from build123d import *
from OCP.BRepFilletAPI import BRepFilletAPI_MakeChamfer

# Parameters (mm, degrees)
EXTRUDE_1_DEPTH      = 1852
FILLET_1_R           = 5
CHAMFER_1_SIZE       = 2
CHAMFER_1_SIZE2      = 1.574468085
EXTRUDE_2_DEPTH      = 822
SKETCH_5_W           = 47
SKETCH_5_H           = 314
EXTRUDE_3_DEPTH      = 30
SKETCH_7_W           = 100
SKETCH_7_H           = 314
CUT_EXTRUDE_1_DEPTH  = 2
SKETCH_8_W           = 23
SKETCH_8_H           = 314
EXTRUDE_4_DEPTH      = 4
SKETCH_9_W           = 48
SKETCH_9_H           = 314
EXTRUDE_5_DEPTH      = 30
SKETCH_10_W          = 100
SKETCH_10_H          = 314
CUT_EXTRUDE_2_DEPTH  = 2
SKETCH_11_W          = 25
SKETCH_11_H          = 314
EXTRUDE_6_DEPTH      = 4
SKETCH_12_W          = 1742
SKETCH_12_H          = 169.004058013
CUT_EXTRUDE_3_DEPTH  = 80
SKETCH_13_W          = 822
SKETCH_13_H          = 239
CUT_EXTRUDE_4_DEPTH  = 5
SKETCH_14_W          = 736
SKETCH_14_H          = 219
CUT_EXTRUDE_5_DEPTH  = 71
SKETCH_15_R          = 45
CUT_EXTRUDE_6_DEPTH  = 1884.868315719
SKETCH_16_W          = 736
SKETCH_16_H          = 41
CUT_EXTRUDE_7_DEPTH  = 20
SKETCH_17_R          = 7.5
CUT_EXTRUDE_8_DEPTH  = 30
SKETCH_18_R          = 7.5
CUT_EXTRUDE_9_DEPTH  = 113
SKETCH_21_R          = 7.5
CUT_EXTRUDE_11_DEPTH = 111
SKETCH_23_R          = 7.5
CUT_EXTRUDE_12_DEPTH = 111


with BuildPart() as part:
    # 草图2 → 凸台-拉伸1 (new body)
    with BuildSketch(Plane(origin=(0, 0, 0), x_dir=(0, 0, -1), z_dir=(1, 0, 0))):
        Polygon((-76.260223553, 62.638496495), (-46.260223553, 62.638496495), (-46.260223553, 27.638496495), (36.739776447, 27.638496495), (36.739776447, -286.361503505), (-46.260223553, -286.361503505), (-46.260223553, -241.361503505), (-41.530493824, -239.739881883), (-43.152115445, -235.010152153), (-76.260223553, -246.361503505), (-76.260223553, -176.361503505), (-66.260223553, -176.361503505), (-66.260223553, -7.357445492), (-71.260223553, -7.357445492), (-71.260223553, -2.361503505), (-76.260223553, -2.361503505), align=None)
    extrude(amount=EXTRUDE_1_DEPTH)

    # 圆角1
    # the kernel refuses this fillet: 5 mm, written as the material it adds along each edge
    with BuildSketch(Plane(origin=(0, -2.361503505, 71.260223553), x_dir=(0, -1, 0), z_dir=(1, 0, 0))) as fillet_1_piece_1_section:
        with BuildLine():
            CenterArc((FILLET_1_R, -FILLET_1_R), FILLET_1_R, 90, 90)
            Line((0, -FILLET_1_R), (0, 0))
            Line((0, 0), (FILLET_1_R, 0))
        make_face()
    fillet_1_piece_1 = extrude(amount=1852, mode=Mode.PRIVATE)
    fillet_1_piece_1 = split(fillet_1_piece_1, bisect_by=Plane(origin=(926, -7.357445492, 72.392274368), z_dir=(0, 1, 0)), keep=Keep.TOP, mode=Mode.PRIVATE)
    add(fillet_1_piece_1)

    # 倒角1: one chamfer whose edges measure the first distance from different faces: ONE call of the kernel's chamfer builder (chamfer() names one face for all edges)
    chamfer_1_edges_1 = [part.edges().sort_by_distance(p)[0] for p in [
        (926, 62.638496495, 76.260223553),
        (926, -286.361503505, 46.260223553),
    ]]
    chamfer_1_edges_2 = [part.edges().sort_by_distance(p)[0] for p in [
        (926, -246.361503505, 76.260223553),
    ]]
    chamfer_1_side_2 = [part.faces().sort_by_distance(p)[0] for p in [
        (926, -211.361503505, 76.260223553),
    ]]
    chamfer_1 = BRepFilletAPI_MakeChamfer(part.part.solid().wrapped)
    for e in chamfer_1_edges_1:
        chamfer_1.Add(CHAMFER_1_SIZE, e.wrapped)
    for e in chamfer_1_edges_2:
        chamfer_1.Add(CHAMFER_1_SIZE, CHAMFER_1_SIZE2, e.wrapped, chamfer_1_side_2[0].wrapped)  # the first distance lies on this face
    add(Compound.cast(chamfer_1.Shape()), mode=Mode.REPLACE)

    # 草图4 → 凸台-拉伸2 (add)
    with BuildSketch(Plane(origin=(1337, 0, 0), x_dir=(0, 0, -1), z_dir=(1, 0, 0))):
        Polygon((36.739776447, 27.638496495), (56.739776447, 27.638496495), (56.739776447, 32.638496495), (71.739776447, 32.638496495), (71.739776447, 67.638496495), (111.739776447, 67.638496495), (111.739776447, -326.361503505), (71.739776447, -326.361503505), (71.739776447, -291.361503505), (56.739776447, -291.361503505), (56.739776447, -286.361503505), (36.739776447, -286.361503505), align=None)
    extrude(amount=-EXTRUDE_2_DEPTH)

    # 草图5 → 凸台-拉伸3 (add)
    with BuildSketch(Plane(origin=(0, 0, -36.739776447), x_dir=(-1, 0, 0), z_dir=(0, 0, -1))):
        with Locations((-1703.5, -129.361503505)):
            Rectangle(SKETCH_5_W, SKETCH_5_H)
    extrude(amount=EXTRUDE_3_DEPTH)

    # 草图7 → 切除-拉伸1 (cut)
    with BuildSketch(Plane(origin=(0, 0, -36.739776447), x_dir=(-1, 0, 0), z_dir=(0, 0, -1))):
        with Locations((-1510, -129.361503505)):
            Rectangle(SKETCH_7_W, SKETCH_7_H)
    extrude(amount=-CUT_EXTRUDE_1_DEPTH, mode=Mode.SUBTRACT)

    # 草图8 → 凸台-拉伸4 (add)
    with BuildSketch(Plane(origin=(0, 0, -36.739776447), x_dir=(-1, 0, 0), z_dir=(0, 0, -1))):
        with Locations((-1348.5, -129.361503505)):
            Rectangle(SKETCH_8_W, SKETCH_8_H)
    extrude(amount=EXTRUDE_4_DEPTH)

    # 草图9 → 凸台-拉伸5 (add)
    with BuildSketch(Plane(origin=(0, 0, -36.739776447), x_dir=(-1, 0, 0), z_dir=(0, 0, -1))):
        with Locations((-136, -129.361503505)):
            Rectangle(SKETCH_9_W, SKETCH_9_H)
    extrude(amount=EXTRUDE_5_DEPTH)

    # 草图10 → 切除-拉伸2 (cut)
    with BuildSketch(Plane(origin=(0, 0, -36.739776447), x_dir=(-1, 0, 0), z_dir=(0, 0, -1))):
        with Locations((-340, -129.361503505)):
            Rectangle(SKETCH_10_W, SKETCH_10_H)
    extrude(amount=-CUT_EXTRUDE_2_DEPTH, mode=Mode.SUBTRACT)

    # 草图11 → 凸台-拉伸6 (add)
    with BuildSketch(Plane(origin=(0, 0, -36.739776447), x_dir=(-1, 0, 0), z_dir=(0, 0, -1))):
        with Locations((-502.5, -129.361503505)):
            Rectangle(SKETCH_11_W, SKETCH_11_H)
    extrude(amount=EXTRUDE_6_DEPTH)

    # 草图12 → 切除-拉伸3 (cut)
    with BuildSketch(Plane.XY.offset(66.260223553)):
        with Locations((926, -91.859474499)):
            Rectangle(SKETCH_12_W, SKETCH_12_H)
    extrude(amount=-CUT_EXTRUDE_3_DEPTH, mode=Mode.SUBTRACT)

    # 草图13 → 切除-拉伸4 (cut)
    with BuildSketch(Plane(origin=(0, 0, -111.739776447), x_dir=(-1, 0, 0), z_dir=(0, 0, -1))):
        with Locations((-926, -125.861503505)):
            Rectangle(SKETCH_13_W, SKETCH_13_H)
    extrude(amount=-CUT_EXTRUDE_4_DEPTH, mode=Mode.SUBTRACT)

    # 草图14 → 切除-拉伸5 (cut)
    with BuildSketch(Plane(origin=(0, 0, -106.739776447), x_dir=(-1, 0, 0), z_dir=(0, 0, -1))):
        with Locations((-926, -125.861503505)):
            Rectangle(SKETCH_14_W, SKETCH_14_H)
    extrude(amount=-CUT_EXTRUDE_5_DEPTH, mode=Mode.SUBTRACT)

    # 草图15 → 切除-拉伸6 (cut, through all)
    with BuildSketch(Plane(origin=(0, 0, -35.739776447), x_dir=(-1, 0, 0), z_dir=(0, 0, -1))):
        with Locations(Location((-1163, -96.361503505, 0), (0, 0, 90))):
            Circle(SKETCH_15_R)
        with Locations(Location((-933, -96.361503505, 0), (0, 0, 90))):
            Circle(SKETCH_15_R)
        with Locations(Location((-703, -96.361503505, 0), (0, 0, 90))):
            Circle(SKETCH_15_R)
        with BuildLine():
            Line((-1226.5, -48.861503505), (-1226.5, -133.861503505))
            ThreePointArc((-1226.5, -133.861503505), (-1239, -146.361503505), (-1251.5, -133.861503505))
            Line((-1251.5, -133.861503505), (-1251.5, -48.861503505))
            ThreePointArc((-1251.5, -48.861503505), (-1239, -36.361503505), (-1226.5, -48.861503505))
        make_face()
    extrude(amount=-CUT_EXTRUDE_6_DEPTH, mode=Mode.SUBTRACT)

    # 草图16 → 切除-拉伸7 (cut)
    with BuildSketch(Plane(origin=(0, -235.361503505, 0), x_dir=(1, 0, 0), z_dir=(0, 1, 0))):
        with Locations((926, 56.239776447)):
            Rectangle(SKETCH_16_W, SKETCH_16_H)
    extrude(amount=-CUT_EXTRUDE_7_DEPTH, mode=Mode.SUBTRACT)

    # 草图17 → 切除-拉伸8 (cut)
    with BuildSketch(Plane(origin=(0, 0, -66.739776447), x_dir=(-1, 0, 0), z_dir=(0, 0, -1))):
        with Locations(Location((-1707, -2.361503505, 0), (0, 0, 90))):
            Circle(SKETCH_17_R)
        with Locations(Location((-1707, -132.361503505, 0), (0, 0, 90))):
            Circle(SKETCH_17_R)
        with Locations(Location((-1707, -262.361503505, 0), (0, 0, 90))):
            Circle(SKETCH_17_R)
        with Locations(Location((-132, -2.361503505, 0), (0, 0, 90))):
            Circle(SKETCH_17_R)
        with Locations(Location((-132, -132.361503505, 0), (0, 0, 90))):
            Circle(SKETCH_17_R)
        with Locations(Location((-132, -262.361503505, 0), (0, 0, 90))):
            Circle(SKETCH_17_R)
    extrude(amount=-CUT_EXTRUDE_8_DEPTH, mode=Mode.SUBTRACT)

    # 草图18 → 切除-拉伸9 (cut)
    with BuildSketch(Plane(origin=(0, 0, -36.739776447), x_dir=(-1, 0, 0), z_dir=(0, 0, -1))):
        with Locations(Location((-1489.500000001, 15.138496495, 0), (0, 0, 90))):
            Circle(SKETCH_18_R)
    extrude(amount=-CUT_EXTRUDE_9_DEPTH, mode=Mode.SUBTRACT)

    # 草图21 → 切除-拉伸11 (cut)
    with BuildSketch(Plane(origin=(0, 0, -34.739776447), x_dir=(-1, 0, 0), z_dir=(0, 0, -1))):
        with Locations(Location((-322.5, 15.138496495, 0), (0, 0, 90))):
            Circle(SKETCH_21_R)
    extrude(amount=-CUT_EXTRUDE_11_DEPTH, mode=Mode.SUBTRACT)

    # 草图23 → 切除-拉伸12 (cut)
    with BuildSketch(Plane(origin=(0, 0, -34.739776447), x_dir=(-1, 0, 0), z_dir=(0, 0, -1))):
        with Locations(Location((-1489.500000001, -204.861503505, 0), (0, 0, 90))):
            Circle(SKETCH_23_R)
        with Locations(Location((-322.5, -204.861503505, 0), (0, 0, 90))):
            Circle(SKETCH_23_R)
    extrude(amount=-CUT_EXTRUDE_12_DEPTH, mode=Mode.SUBTRACT)


solid = part.part
Here's how the part is built. I have some questions about the finished solid (model axes, mm). A direction names the side the tool comes from. Coordinates: 2 decimals unless noted, no trailing zeros. Loops run counter-clockwise (first coordinate to the right, second up) from the corner with the lowest first, then second, coordinate; pieces in that order, holes last.
1. For P1, Ø13.5, axis at x = 1489.5, y = -204.86, coming from the +Z side; P2, Ø3, axis at x = 995.5, z = -40, coming from the +Y side; P3, Ø14, axis at x = 1706.5, y = -70.5, coming from the -Z side; P4, Ø5, axis at x = 585, y = -19, coming from the -Z side, each with a flat end and sliding along its axis, tell me the tip position at first contact or that it passes through.
2. Imagine slicing it at B-B, the plane z = 9.5. Please give me the cut outline in (x, y), and give its area (3 significant figures).
3. I need wall thicknesses on L1, parallel to X at y = -1, z = -43; L2, parallel to Y at x = 1707, z = -46; L3, parallel to X at y = 17, z = 57. Which ranges of each line are inside material? Lowest first, please.
4. If we mould it in two halves opening along Y, with no side actions, what happens to faces 4 (the flat face through (921, -255.362, -57)), 5 (the cylindrical face through (747.617, -102.22, -24.894)), 6 (the flat face through (1699, -127, -66.74))? For each: pulls with the +Y half, pulls with the -Y half, needs draft (parallel to the pull), parting line crosses it, or undercut.
5. For faces 1 (the flat face through (958, -240, -106.74)), 2 (the flat face through (224, -127, -36.74)), 3 (the flat face through (913, -176.362, 32)), which set-ups out of +Z, -Z, +X, -X, +Y, -Y let a thin tool reach every point of the face, with its end or its side?
6. Imagine slicing it at A-A, the plane x = 1425. Please give me the cut outline in (y, z).
7. Imagine slicing it at C-C, the plane y = -94. Count the separate pieces of the cut face and the enclosed holes in it, and give its area (3 significant figures).
Taken from the geometry:
1. P1: passes through
1. P2: stops at y = 27.64
1. P3: stops at z = -66.74
1. P4: stops at z = -35.74
2. outline: (0, -286.36) - (1852, -286.36) - (1852, 27.64) - (0, 27.64) - close; hole (55, -176.36) - (1797, -176.36) - (1797, -7.36) - (55, -7.36) - close; hole circle Ø15 at (322.5, -204.86); hole circle Ø15 at (322.5, 15.14); hole circle Ø15 at (1489.5, -204.86); hole circle Ø15 at (1489.5, 15.14)
2. area: 286,000 mm2
3. L1: x = 112 to 124.62, 139.38 to 160, 515 to 1337, 1680 to 1699.62, 1714.38 to 1727
3. L2: y = -286.36 to -269.86, -254.86 to -139.86, -124.86 to -9.86, 5.14 to 27.64
3. L3: x = 0 to 315.23, 329.77 to 1482.23, 1496.77 to 1852
4. face 4: undercut
4. face 5: undercut
4. face 6: needs draft
5. face 1: -Z, +X, -X
5. face 2: -Z, +Y, -Y
5. face 3: +Z
6. outline: (-286.36, -36.74) - (27.64, -36.74) - (27.64, 46.26) - (62.64, 46.26) - (62.64, 74.26) - (60.64, 76.26) - (-2.36, 76.26) arc R5 cw to (-7.36, 71.26) - (-7.36, -13.74) - (-176.36, -13.74) - (-176.36, 76.26) - (-244.36, 76.26) - (-245.85, 74.77) - (-235.01, 43.15) - (-239.74, 41.53) - (-241.36, 46.26) - (-284.36, 46.26) - (-286.36, 44.26) - close
7. separate pieces: 5
7. enclosed holes: 0
7. area: 52,800 mm2
